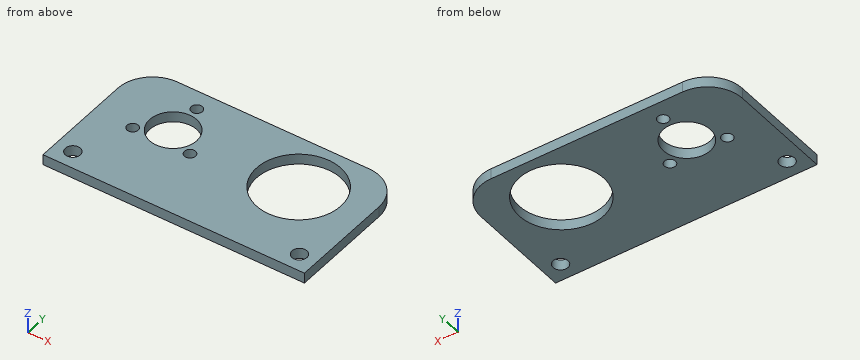
from build123d import *

# Parameters (mm, degrees)
SKETCH_1_W      = 75
SKETCH_1_H      = 40
SKETCH_1_R      = 6.75
SKETCH_1_R_2    = 1.6
SKETCH_1_R_3    = 12.1
SKETCH_1_R_4    = 2.15
EXTRUDE_1_DEPTH = 3
FILLET_1_R      = 10


with BuildPart() as part:
    # ｽｹｯﾁ1 → ﾎﾞｽ - 押し出し1 (new body)
    with BuildSketch(Plane.XY):
        with Locations((37.5, 20)):
            Rectangle(SKETCH_1_W, SKETCH_1_H)
        with Locations((19.5, 25)):
            Circle(SKETCH_1_R, mode=Mode.SUBTRACT)
        with Locations((19.5, 34.5)):
            Circle(SKETCH_1_R_2, mode=Mode.SUBTRACT)
        with Locations((27.727241336, 20.25)):
            Circle(SKETCH_1_R_2, mode=Mode.SUBTRACT)
        with Locations((11.272758664, 20.25)):
            Circle(SKETCH_1_R_2, mode=Mode.SUBTRACT)
        with Locations((55.5, 25)):
            Circle(SKETCH_1_R_3, mode=Mode.SUBTRACT)
        with Locations((5, 5)):
            Circle(SKETCH_1_R_4, mode=Mode.SUBTRACT)
        with Locations(Location((70, 5, 0), (0, 0, 180))):
            Circle(SKETCH_1_R_4, mode=Mode.SUBTRACT)
    extrude(amount=EXTRUDE_1_DEPTH)

    # ﾌｨﾚｯﾄ1
    fillet_1_edges = [part.edges().sort_by_distance(p)[0] for p in [
        (0, 40, 1.5),
        (75, 40, 1.5),
    ]]
    fillet(fillet_1_edges, radius=FILLET_1_R)


solid = part.part
Design review of the part built by this model. Coordinates are the model's own, in mm. Round coordinates to 2 decimals unless told otherwise and drop trailing zeros. Write each loop counter-clockwise with the first axis right and the second up, starting at its lowest first coordinate (ties: lowest second). Pieces come first, ordered by that corner, then holes. Notation, with made-up numbers: (-34.75, 9.5) -> (3.25, 9.5) arc R14 ccw to (3.25, 30.5) -> close; hole circle Ø3 at (-19, 85). An arc over 180 degrees is marked (long way). One line per question, with ' | ' between items.
(1) Take a section at A-A, the plane x = 19.5. State the section outline as (y, z) points, and give its area (3 significant figures).
Result sheet:
outline: (0, 0) -> (18.25, 0) -> (18.25, 3) -> (0, 3) -> close; (31.75, 0) -> (32.9, 0) -> (32.9, 3) -> (31.75, 3) -> close; (36.1, 0) -> (40, 0) -> (40, 3) -> (36.1, 3) -> close | area: 69.9 mm2
(2) Take a section at C-C, the plane x = 55.5. State the section outline as (y, z) points.
Result sheet:
outline: (0, 0) -> (12.9, 0) -> (12.9, 3) -> (0, 3) -> close; (37.1, 0) -> (40, 0) -> (40, 3) -> (37.1, 3) -> close
(3) Take a section at D-D, the plane z = 1.05. State the section outline as (x, y) points, and give its area (3 significant figures).
Result sheet:
outline: (0, 0) -> (75, 0) -> (75, 30) arc R10 ccw to (65, 40) -> (10, 40) arc R10 ccw to (0, 30) -> close; hole circle Ø4.3 at (5, 5); hole circle Ø3.2 at (11.27, 20.25); hole circle Ø13.5 at (19.5, 25); hole circle Ø3.2 at (19.5, 34.5); hole circle Ø3.2 at (27.73, 20.25); hole circle Ø24.2 at (55.5, 25); hole circle Ø4.3 at (70, 5) | area: 2,300 mm2
(4) Wall thickness on line 1 (Y direction, x = 19.5, z = 2.4); line 2 (Y direction, x = 55.5, z = 1.65); line 3 (X direction, y = 6.5, z = 2.5): over which ranges is each line inside the solid? List them lowest first. Write a range as [from, to].
Result sheet:
line 1: [0, 18.25], [31.75, 32.9], [36.1, 40] | line 2: [0, 12.9], [37.1, 40] | line 3: [0, 3.46], [6.54, 68.46], [71.54, 75]
(5) Take a section at B-B, the plane y = 25. State the section outline as (x, z) points.
Result sheet:
outline: (0, 0) -> (12.75, 0) -> (12.75, 3) -> (0, 3) -> close; (26.25, 0) -> (43.4, 0) -> (43.4, 3) -> (26.25, 3) -> close; (67.6, 0) -> (75, 0) -> (75, 3) -> (67.6, 3) -> close
